from build123d import *

# Parameters (mm, degrees)
SKETCH1_R           = 3.795
BOSS_EXTRUDE1_DEPTH = 20
SKETCH2_W           = 30
SKETCH2_H           = 30
BOSS_EXTRUDE2_DEPTH = 10


with BuildPart() as part:
    # Sketch1 → Boss-Extrude1 (new body)
    with BuildSketch(Plane.XY):
        with Locations((126.972995011, 125.730606971)):
            Circle(SKETCH1_R)
    extrude(amount=-BOSS_EXTRUDE1_DEPTH)

    # Sketch2 → Boss-Extrude2 (add)
    with BuildSketch(Plane.XY):
        with Locations((126.972995011, 125.730606971)):
            Rectangle(SKETCH2_W, SKETCH2_H)
    extrude(amount=BOSS_EXTRUDE2_DEPTH)

    # Sketch3 → Revolve1 (revolve)
    with BuildSketch(Plane(origin=(126.972995011, 0, 0), x_dir=(0, 0, -1), z_dir=(1, 0, 0))):
        Polygon((-0.758524561, 110.730606971), (-5, 90.117115807), (-5, 110.730606971), align=None)
    revolve(axis=Axis((126.972995011, 90.117115807, 5), (0, 1, 0)))


solid = part.part
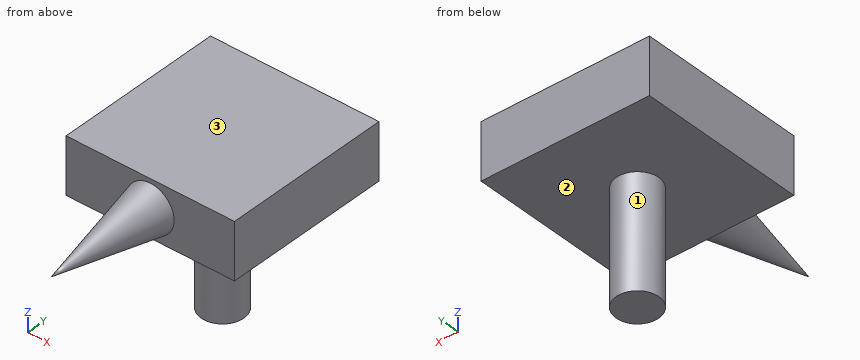
For this review, take the finished solid that the model builds, in its own axes (mm). Face numbers are marked on the shaded views. Round coordinates to 2 decimals unless told otherwise and drop trailing zeros. Write each loop counter-clockwise with the first axis right and the second up, starting at its lowest first coordinate (ties: lowest second). Pieces come first, ordered by that corner, then holes. Notation, with made-up numbers: M -35,51.5 L 8,51.5 A19 cw 8,64.5 Z; hole C 45,48.25 d3. An arc over 180 degrees is marked long. Write item = value, one per line. Start each with the question number.
(1) We need section D-D (y = 127). Give the boundary of the cut face in (x, z), then the cut area to 3 significant figures.
(2) The part is to be moulded in two halves that separate along Z. For the marked faces 1, 2 and 3, say which applies: +Z half, -Z half, draft (parallel to the pull), parting line (faces both ways), or undercut.
(3) We need section C-C (z = -5.25). Give the boundary of the cut face in (x, y) (3 decimals).
(4) Clearance check with flat-ended pins moving along their axes: pin 1 Ø2 at (x, z) = (124.5, -9) entering from +Y; pin 2 Ø10 at (x, y) = (130, 99.5) entering from +Z; pin 3 Ø8 at (x, y) = (132, 106.5) entering from -Z. State where each tip first meets the part, or that it passes through.
(5) We need section B-B (x = 115.5). Give the boundary of the cut face in (y, z), then the cut area to 3 significant figures.
(6) For line 1 along Z through (x, y) = (120, 129); line 2 along Y through (x, z) = (140.75, 6.5); line 3 along Y through (x, z) = (124, -2.5), list the stretches that pass through material, from the lowest coordinate up.
(7) We need section A-A (y = 132.5). Give the boundary of the cut face in (x, z), then the cut area to 3 significant figures.
Results found:
q1.outline = M 111.97,0 L 123.4,0 L 123.4,-20 L 130.55,-20 L 130.55,0 L 141.97,0 L 141.97,10 L 111.97,10 Z
q1.area = 443 mm²
q2.face_1 = draft
q2.face_2 = -Z half
q2.face_3 = +Z half
q3.outline = C 126.973,125.731 d7.59
q4.pin_1 = 129.23
q4.pin_2 = 7.78
q4.pin_3 = 1.55
q5.outline = M 110.73,0 L 140.73,0 L 140.73,10 L 110.73,10 Z
q5.area = 300 mm²
q6.line_1 = 0 to 10
q6.line_2 = 110.73 to 140.73
q6.line_3 = 123.37 to 128.09
q7.outline = M 111.97,0 L 141.97,0 L 141.97,10 L 111.97,10 Z
q7.area = 300 mm²
